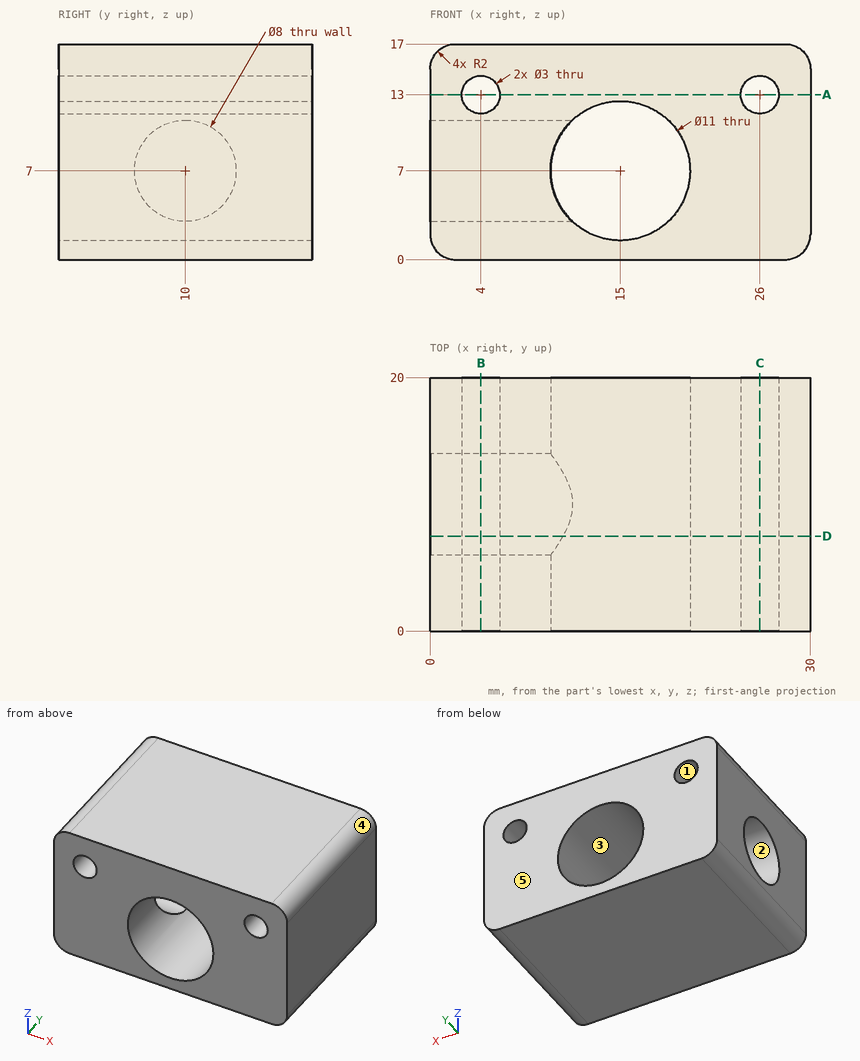
Study the drawing (mm; zero at the part's minimum x, y, z) and answer. A direction names the side the tool comes from. Round coordinates to 2 decimals unless told otherwise and drop trailing zeros. Write each loop counter-clockwise with the first axis right and the second up, starting at its lowest first coordinate (ties: lowest second). Pieces come first, ordered by that corner, then holes. Notation, with made-up numbers: (86.25, -19.75) - (94.25, -19.75) arc R22 ccw to (94.25, -3.75) - close; hole circle Ø5 at (-23, 73.25). An arc over 180 degrees is marked (long way). Return JSON: item names as keys, results as strings. Group by question number.
Q1. For the marked faces 1 and 2, determine the directions among +Z, -Z, +X, -X, +Y, -Y from which every point of the face is accessible in a straight line to the end or side of a thin tool.
Q2. The part is cut by section D-D on y = 7.5. Write down the section's boundary in (x, z).
Q3. The part is cut by section B-B on x = 4. Write down the section's boundary in (y, z), then the cut area to 3 significant figures.
Q4. The part is cut by section A-A on z = 13. Write down the section's boundary in (x, y).
Q5. The mould has two halves that part along Z. Classify the marked faces 3, 4 and 5: released by +Z, released by -Z, zero draft, split by the parting line, or undercut.
Q6. The part is cut by section C-C on x = 26. Write down the section's boundary in (y, z), then the cut area to 3 significant figures.
Q7. Find the intervals of material crossed by L1, parallel to Y at x = 6.5, z = 7; L2, parallel to X at y = 5.5, z = 13.25; L3, parallel to X at y = 5, z = 7, in increasing order.
Solved:
{
 "1": {"face 1": "+Y, -Y", "face 2": "-X"},
 "2": {"outline": "(0, 2) arc R2 ccw to (2, 0) - (28, 0) arc R2 ccw to (30, 2) - (30, 15) arc R2 ccw to (28, 17) - (2, 17) arc R2 ccw to (0, 15) - (0, 10.12) - (10.47, 10.12) arc R5.5 cw (long way) to (10.47, 3.88) - (0, 3.88) - close; hole circle Ø3 at (4, 13); hole circle Ø3 at (26, 13)"},
 "3": {"outline": "(0, 0) - (20, 0) - (20, 11.5) - (0, 11.5) - close; (0, 14.5) - (20, 14.5) - (20, 17) - (0, 17) - close; hole circle Ø8 at (10, 7)", "area": "230 mm²"},
 "4": {"outline": "(0, 0) - (2.5, 0) - (2.5, 20) - (0, 20) - close; (5.5, 0) - (24.5, 0) - (24.5, 20) - (5.5, 20) - close; (27.5, 0) - (30, 0) - (30, 20) - (27.5, 20) - close"},
 "5": {"face 3": "undercut", "face 4": "released by +Z", "face 5": "zero draft"},
 "6": {"outline": "(0, 0) - (20, 0) - (20, 11.5) - (0, 11.5) - close; (0, 14.5) - (20, 14.5) - (20, 17) - (0, 17) - close", "area": "280 mm²"},
 "7": {"L1": "0 to 6, 14 to 20", "L2": "0 to 2.52, 5.48 to 24.52, 27.48 to 30", "L3": "0 to 9.5, 20.5 to 30"}
}
